Work out the finished part from the listing and answer in its coordinate system (mm). A direction names the side the tool comes from. Coordinates: 2 decimals unless noted, no trailing zeros. Loops run counter-clockwise (first coordinate to the right, second up) from the corner with the lowest first, then second, coordinate; pieces in that order, holes last.
```python
from build123d import *

# Parameters (mm, degrees)
F_12_0MM_DOWEL_HOLE1_D = 12
CIRPATTERN1_COUNT      = 4


with BuildPart() as part:
    # Sketch1 → Revolve1 (revolve)
    with BuildSketch(Plane.XY, mode=Mode.PRIVATE) as revolve1_sk:
        with BuildLine():
            Line((-60, 0), (-60, 16))
            Line((-60, 16), (-31, 16))
            ThreePointArc((-31, 16), (-28.878679656, 16.878679656), (-28, 19))
            Line((-28, 19), (-28, 32))
            Line((-28, 32), (-10, 32))
            Line((-10, 32), (-10, 12))
            Line((-10, 12), (-23, 12))
            Line((-23, 12), (-23, 0))
            Line((-23, 0), (-60, 0))
        make_face()
    revolve(revolve1_sk.sketch.rotate(Axis((0, 0, 0), (0, 1, 0)), 270), axis=Axis((0, 0, 0), (0, 1, 0)))

    # Ø12.0mm Dowel Hole1 (through all)
    with Locations(Plane.XZ):
        with Locations((0, 42)):
            f_12_0mm_dowel_hole1 = Hole(F_12_0MM_DOWEL_HOLE1_D / 2)

    # CirPattern1: Ø12.0mm Dowel Hole1 ×4 about axis
    cirpattern1_axis = Axis((0, 0, 0), (0, 1, 0))
    for i in range(1, CIRPATTERN1_COUNT):
        add(f_12_0mm_dowel_hole1.rotate(cirpattern1_axis, i * 360 / CIRPATTERN1_COUNT), mode=Mode.SUBTRACT)


solid = part.part
```
1. Straight lines are drawn through the part: probe 1 along X at (y, z) = (5, 0); probe 2 along Y at (x, z) = (44, 27.5); probe 3 along Z at (x, y) = (5.5, 3.5). For each, find the intervals that lie inside material, in ascending order.
2. A cutting plane is placed at C-C, the plane y = 25. Give the vertices of the cut face in (x, z).
3. A cutting plane is placed at D-D, the plane x = -42. Give the vertices of the cut face in (y, z), then the cut area to 3 significant figures.
4. A cutting plane is placed at B-B, the plane x = 0. Give the vertices of the cut face in (y, z).
5. A cutting plane is placed at A-A, the plane z = 0. Give the vertices of the cut face in (x, y).
6. Determine the mould class of faces 3 (the flat face through (26, 16, -26)), 4 (the cylindrical face through (-42, 8, 6)), 5 (the cylindrical face through (27.334, 25.591, 6.07)) for opening direction X: released by +X, released by -X, zero draft, split by the parting line, or undercut.
7. For faces 1 (the flat face through (5, 12, 10)), 2 (the cylindrical face through (-2.64, 8.11, 59.94)), determine the directions among +Z, -Z, +X, -X, +Y, -Y from which every point of the face is accessible in a straight line to the end or side of a thin tool.
8. Each of these flat-tipped pins is pushed along its axis until it touches: P1, Ø8, axis at y = 26, z = 27, coming from the -X side; P2, Ø12, axis at x = -4, z = -40.5, coming from the +Y side; P3, Ø1, axis at x = 9.5, y = 3.5, coming from the +Z side. Where does it stop, or does it pass through?
Answers below:
1. probe 1: x = -60 to -48, -36 to -23, 23 to 36, 48 to 60
1. probe 2: y = 0 to 16
1. probe 3: z = -59.75 to -44.4, -39.6 to -22.33, 22.33 to 39.6, 44.4 to 59.75
2. outline: circle Ø56 at (0, 0); hole circle Ø20 at (0, 0)
3. outline: (0, -42.85) - (16, -42.85) - (16, -6) - (0, -6) - close; (0, 6) - (16, 6) - (16, 42.85) - (0, 42.85) - close
3. area: 1,180 mm2
4. outline: (0, -60) - (16, -60) - (16, -48) - (0, -48) - close; (0, -36) - (16, -36) - (16, -31) arc R3 cw to (19, -28) - (32, -28) - (32, -10) - (12, -10) - (12, -23) - (0, -23) - close; (0, 23) - (12, 23) - (12, 10) - (32, 10) - (32, 28) - (19, 28) arc R3 cw to (16, 31) - (16, 36) - (0, 36) - close; (0, 48) - (16, 48) - (16, 60) - (0, 60) - close
5. outline: (-60, 0) - (-48, 0) - (-48, 16) - (-60, 16) - close; (-36, 0) - (-23, 0) - (-23, 12) - (-10, 12) - (-10, 32) - (-28, 32) - (-28, 19) arc R3 cw to (-31, 16) - (-36, 16) - close; (10, 12) - (23, 12) - (23, 0) - (36, 0) - (36, 16) - (31, 16) arc R3 cw to (28, 19) - (28, 32) - (10, 32) - close; (48, 0) - (60, 0) - (60, 16) - (48, 16) - close
6. face 3: zero draft
6. face 4: undercut
6. face 5: split by the parting line
7. face 1: -Y
7. face 2: +Y, -Y
8. P1: stops at x = -15.97
8. P2: stops at y = 16
8. P3: stops at z = 59.32
